```python
from build123d import *

# Parameters (mm, degrees)
F0_R     = 1.5098129389
F0_R_2   = 1.5
F1_DEPTH = 6


# Not quite as in the source:
# - ends of sketch curves that miss each other by under 0.0002 mm in the source are joined


with BuildPart() as f1:
    # F0 (on Top) → F1 (new body)
    with BuildSketch(Plane.XY):
        with BuildLine():
            Line((4.5e-05, 95.32702), (-83.6431340024, 95.32702))
            Line((-83.6431340024, 95.32702), (-98.2850169252, 109.9708148351))
            Line((-98.2850169252, 109.9708148351), (-99.0283260424, 110.7142210123))
            ThreePointArc((-99.0283260424, 110.7142210123), (-110.2653878227, 110.4426468905), (-110.8769341282, 99.2189522637))
            Line((-110.8769341282, 99.2189522637), (-97.25943, 85.599669985))
            Line((-97.25943, 85.599669985), (-97.25943, -2.5e-06))
            Line((-97.25943, -2.5e-06), (-97.2594255995, -85.5996749849))
            Line((-97.2594255995, -85.5996749849), (-110.8769290275, -99.2189579637))
            ThreePointArc((-110.8769290275, -99.2189579637), (-110.2653821451, -110.4426525591), (-99.0283203508, -110.7142261032))
            Line((-99.0283203508, -110.7142261032), (-98.2850112718, -109.9708198877))
            Line((-98.2850112718, -109.9708198877), (-83.6431291018, -95.3270243))
            Line((-83.6431291018, -95.3270243), (4.99006e-05, -95.32702))
            Line((4.99006e-05, -95.32702), (83.6432191018, -95.3270243))
            Line((83.6432191018, -95.3270243), (98.2851012718, -109.9708198877))
            Line((98.2851012718, -109.9708198877), (99.0284103508, -110.7142261032))
            ThreePointArc((99.0284103508, -110.7142261032), (110.2654721451, -110.4426525591), (110.8770190275, -99.2189579637))
            Line((110.8770190275, -99.2189579637), (97.2595155995, -85.5996749849))
            Line((97.2595155995, -85.5996749849), (97.25952, -2.5e-06))
            Line((97.25952, -2.5e-06), (97.25952, 85.599669985))
            Line((97.25952, 85.599669985), (110.8770241282, 99.2189522637))
            ThreePointArc((110.8770241282, 99.2189522637), (110.2654778227, 110.4426468905), (99.0284160424, 110.7142210123))
            Line((99.0284160424, 110.7142210123), (98.2851069252, 109.9708148351))
            Line((98.2851069252, 109.9708148351), (83.6432240024, 95.32702))
            Line((83.6432240024, 95.32702), (4.5e-05, 95.32702))
        make_face()
        with Locations((-104.4999496278, -104.5000026861)):
            Circle(F0_R, mode=Mode.SUBTRACT)
        with Locations((-73.0099637148, -25.0000018767)):
            Circle(F0_R_2, mode=Mode.SUBTRACT)
        with Locations((104.5000396278, -104.5000026861)):
            Circle(F0_R, mode=Mode.SUBTRACT)
        with Locations((73.0100537148, -25.0000018767)):
            Circle(F0_R_2, mode=Mode.SUBTRACT)
        with Locations((-73.009965, 24.9999981233)):
            Circle(F0_R_2, mode=Mode.SUBTRACT)
        with Locations((-104.499955, 104.4999973139)):
            Circle(F0_R, mode=Mode.SUBTRACT)
        with Locations((73.010055, 24.9999981233)):
            Circle(F0_R_2, mode=Mode.SUBTRACT)
        with Locations((104.500045, 104.4999973139)):
            Circle(F0_R, mode=Mode.SUBTRACT)
        with BuildLine():
            Line((-99.0283260424, 110.7142210123), (-98.2850169252, 109.9708148351))
            ThreePointArc((-98.2850169252, 109.9708148351), (-98.6448610267, 110.3543268389), (-99.0283260424, 110.7142210123))
        make_face()
        with BuildLine():
            ThreePointArc((99.0284160424, 110.7142210123), (98.6449510267, 110.3543268389), (98.2851069252, 109.9708148351))
            Line((98.2851069252, 109.9708148351), (99.0284160424, 110.7142210123))
        make_face()
        with BuildLine():
            Line((-98.2850112718, -109.9708198877), (-99.0283203508, -110.7142261032))
            ThreePointArc((-99.0283203508, -110.7142261032), (-98.6448553535, -110.35433191), (-98.2850112718, -109.9708198877))
        make_face()
        with BuildLine():
            ThreePointArc((98.2851012718, -109.9708198877), (98.6449453535, -110.35433191), (99.0284103508, -110.7142261032))
            Line((99.0284103508, -110.7142261032), (98.2851012718, -109.9708198877))
        make_face()
    extrude(amount=F1_DEPTH)


solid = f1.part
```
The model under review builds one solid part; all positions refer to its coordinate system, in mm. A direction names the side the tool comes from. Round coordinates to 2 decimals unless told otherwise and drop trailing zeros. Loops run counter-clockwise (first coordinate to the right, second up) from the corner with the lowest first, then second, coordinate; pieces in that order, holes last. Notation, with made-up numbers: (60, -38.75) -> (113, -38.75) arc R5 ccw to (113, -34.75) -> close; hole circle Ø7 at (50, -23). An arc over 180 degrees is marked (long way). Answer in a Markdown table with one row per item.
1) Consider section C-C, the plane y = -34.5. Write out the cut boundary in (x, z), plus the area to 3 significant figures.
Taken from the geometry:
| item | result |
|---|---|
| outline | (-97.26, 0) -> (97.26, 0) -> (97.26, 6) -> (-97.26, 6) -> close |
| area | 1,170 mm² |
2) Consider section B-B, the plane x = -27.5. Write out the cut boundary in (y, z).
Taken from the geometry:
| item | result |
|---|---|
| outline | (-95.33, 0) -> (95.33, 0) -> (95.33, 6) -> (-95.33, 6) -> close |
3) Draft analysis for pull direction Y (two halves, no side actions). For faces 1 (the flat face through (104.16, -92.5, 2.96)), 2 (the flat face through (-104.16, 92.5, 2.96)), 3 (the flat face through (1, 95.327, 3)), 4 (the flat face through (-2, 2, 0)), state which applies: pulls with the +Y half, pulls with the -Y half, needs draft (parallel to the pull), parting line crosses it, or undercut.
Taken from the geometry:
| item | result |
|---|---|
| face 1 | undercut |
| face 2 | undercut |
| face 3 | pulls with the +Y half |
| face 4 | needs draft |
4) Tool access review of faces 5 (the flat face through (90.862, -102.546, 2.958)), 6 (the flat face through (-103.97, -92.31, 2.96)), 7 (the flat face through (-90.862, 102.546, 2.958)): name each direction out of +Z, -Z, +X, -X, +Y, -Y from which nothing blocks a thin tool from reaching the whole face with its end or side.
Taken from the geometry:
| item | result |
|---|---|
| face 5 | +Z, -Z, -Y |
| face 6 | +Z, -Z, -X |
| face 7 | +Z, -Z, +Y |
5) For pin 1 Ø1.8 at (y, z) = (44.5, 4) entering from -X; pin 2 Ø2 at (x, z) = (85, 1) entering from +Y; pin 3 Ø3 at (y, z) = (50.5, 4) entering from +X, all flat-tipped, find the tip position at first contact; note any pin that passes through.
Taken from the geometry:
| item | result |
|---|---|
| pin 1 | stops at x = -97.26 |
| pin 2 | stops at y = 97.68 |
| pin 3 | stops at x = 97.26 |
6) Wall thickness on line 1 along X through (y, z) = (104, 4.5); line 2 along Y through (x, z) = (-8.5, 5.45); line 3 along Y through (x, z) = (-97.5, 0.5): over which ranges is each line inside the solid? List them lowest first.
Taken from the geometry:
| item | result |
|---|---|
| line 1 | x = -112.76 to -105.92, -103.08 to -92.31, 92.32 to 103.08, 105.92 to 112.76 |
| line 2 | y = -95.33 to 95.33 |
| line 3 | y = -109.19 to -85.84, 85.84 to 109.19 |
7) Consider section A-A, the plane z = 2.6. Count the separate pieces of the cut face and the enclosed holes in it, plus the area to 3 significant figures.
Taken from the geometry:
| item | result |
|---|---|
| separate pieces | 1 |
| enclosed holes | 8 |
| area | 38,500 mm² |
